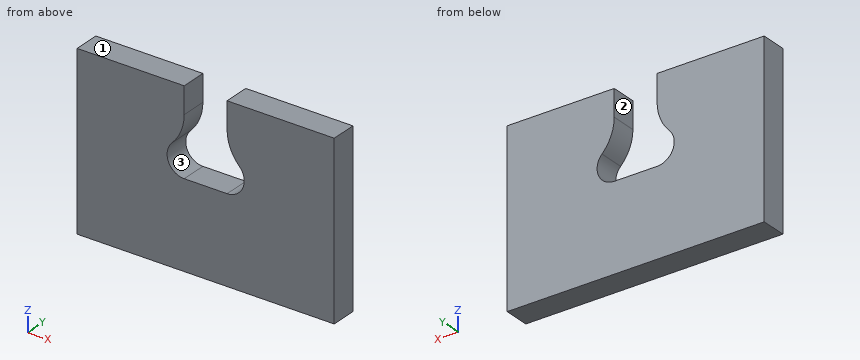
```python
from build123d import *

# Parameters (mm, degrees)
BOSS_EXTRUDE1_DEPTH = 3


with BuildPart() as part:
    # Sketch1 → Boss-Extrude1 (new body)
    with BuildSketch(Plane(origin=(0, 0, 0), x_dir=(1, 0, 0), z_dir=(0, 1, 0))):
        with BuildLine():
            Line((-2.5, 0), (-2.5, 3.101020514))
            ThreePointArc((-2.5, 3.101020514), (-2.870899501, 4.990842879), (-3.928571429, 6.600291576))
            ThreePointArc((-3.928571429, 6.600291576), (-4.343829825, 8.774784858), (-2.5, 10))
            Line((-2.5, 10), (2.5, 10))
            ThreePointArc((2.5, 10), (4.343829825, 8.774784858), (3.928571429, 6.600291576))
            ThreePointArc((3.928571429, 6.600291576), (2.870899501, 4.990842879), (2.5, 3.101020514))
            Line((2.5, 3.101020514), (2.5, 0))
            Line((2.5, 0), (15, 0))
            Line((15, 0), (15, 20))
            Line((15, 20), (-15, 20))
            Line((-15, 20), (-15, 0))
            Line((-15, 0), (-2.5, 0))
        make_face()
    extrude(amount=BOSS_EXTRUDE1_DEPTH)


solid = part.part
```
Geometry: final body of the model. Coordinates: model frame, mm. Face numbers are marked on the shaded views. A direction names the side the tool comes from. Give positions to 0.01 mm unless a question says otherwise; leave off trailing zeros. Loops run counter-clockwise (first coordinate to the right, second up) from the corner with the lowest first, then second, coordinate; pieces in that order, holes last. Notation, with made-up numbers: (-31.75, -11) -> (-21.75, -11) arc R36 cw to (-21.75, 26) -> close; hole circle Ø6 at (48.5, 1). An arc over 180 degrees is marked (long way). Use one line per item in the form item = value.
Item 1: Section query A-A on z = -2.5. Output: boundary loops of the cut face in (x, y), and give its area (3 significant figures).
A:
outline = (-15, 0) -> (-2.5, 0) -> (-2.5, 3) -> (-15, 3) -> close; (2.5, 0) -> (15, 0) -> (15, 3) -> (2.5, 3) -> close
area = 75.0 mm^2
Item 2: Section query C-C on z = -7.25. Output: boundary loops of the cut face in (x, y), and give its area (3 significant figures).
A:
outline = (-15, 0) -> (-4.35, 0) -> (-4.35, 3) -> (-15, 3) -> close; (4.35, 0) -> (15, 0) -> (15, 3) -> (4.35, 3) -> close
area = 63.9 mm^2
Item 3: Pin query (flat end, axial travel): P1, Ø0.9, axis at x = 0, y = 1.5, coming from the +Z side. Return the tip coordinate at first contact, or that it passes through.
A:
P1 = -10
Item 4: Access query for the marked faces 1, 2 and 3. Directions: +Z, -Z, +X, -X, +Y, -Y. A direction counts if a zero-diameter tool reaches every point of the face in a straight line with its end or side. Return the directions, or none.
A:
face_1 = +Z, +X, -X, +Y, -Y
face_2 = +Z, +Y, -Y
face_3 = +Y, -Y
Item 5: Line query: probe 1 along X at (y, z) = (0.95, -8); probe 2 along X at (y, z) = (2.3, -3.25); probe 3 along Z at (x, y) = (-1.75, 1.25). Output: solid intervals per line, ascending.
A:
probe_1 = -15 to -4.5, 4.5 to 15
probe_2 = -15 to -2.5, 2.5 to 15
probe_3 = -20 to -10
Item 6: Section query D-D on x = -1. Output: boundary loops of the cut face in (y, z).
A:
outline = (0, -20) -> (3, -20) -> (3, -10) -> (0, -10) -> close
Item 7: Section query B-B on y = 1.35. Output: boundary loops of the cut face in (x, z).
A:
outline = (-15, -20) -> (15, -20) -> (15, 0) -> (2.5, 0) -> (2.5, -3.1) arc R5 ccw to (3.93, -6.6) arc R2 cw to (2.5, -10) -> (-2.5, -10) arc R2 cw to (-3.93, -6.6) arc R5 ccw to (-2.5, -3.1) -> (-2.5, 0) -> (-15, 0) -> close
